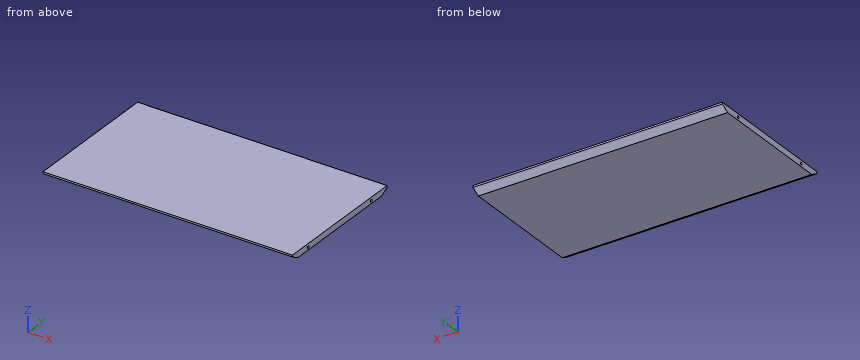
```python
from build123d import *

# Parameters (mm, degrees)
F0_W           = 800
F0_H           = 450
F1_DEPTH       = 20
F3_START       = -400.001
F3_DEPTH       = 800.002
F6_D           = 8
F6_DEPTH       = 30
F6_TIP         = 2.4034424761
F6_ON_F5_D     = 8
F6_ON_F5_DEPTH = 30
F6_ON_F5_TIP   = 2.4034424761


with BuildPart() as f1:
    # F0 (on Top) → F1 (new body)
    with BuildSketch(Plane.XY):
        Rectangle(F0_W, F0_H)
    extrude(amount=F1_DEPTH)

    # F2 (on Right) → F3 (intersect)
    with BuildSketch(Plane.YZ.offset(F3_START)):
        Polygon((-200, 0), (200, 0), (234.6410161514, 20), (-234.6410161514, 20), align=None)
    extrude(amount=F3_DEPTH, mode=Mode.INTERSECT)

    # F6
    with Locations(Plane(origin=(-400, 0, 0), x_dir=(0, -1, 0), z_dir=(-1, 0, 0))):
        with Locations((-150, 9), (150, 9)):
            Hole(F6_D / 2, depth=F6_DEPTH)
            with Locations((0, 0, -(F6_DEPTH + F6_TIP / 2))):  # 118° drill point
                Cone(0, F6_D / 2, F6_TIP, mode=Mode.SUBTRACT)

    # F6 on F5
    with Locations(Plane.YZ.offset(400)):
        with Locations((150, 9), (-150, 9)):
            Hole(F6_ON_F5_D / 2, depth=F6_ON_F5_DEPTH)
            with Locations((0, 0, -(F6_ON_F5_DEPTH + F6_ON_F5_TIP / 2))):  # 118° drill point
                Cone(0, F6_ON_F5_D / 2, F6_ON_F5_TIP, mode=Mode.SUBTRACT)


solid = f1.part
```
Verification items for the finished model (mm, model axes). Round coordinates to 2 decimals unless told otherwise and drop trailing zeros. Loops run counter-clockwise (first coordinate to the right, second up) from the corner with the lowest first, then second, coordinate; pieces in that order, holes last. Notation, with made-up numbers: (-16.75, 80) -> (39.25, 80) arc R13 cw to (39.25, 89) -> close; hole circle Ø5 at (47.5, -29). An arc over 180 degrees is marked (long way). Answer as a JSON object with one key per item and string values.
Q1. Section check A-A (x = 82.5). Record the boundary of the cut face in (y, z).
Data:
{"outline": "(-225, 14.43) -> (-200, 0) -> (200, 0) -> (225, 14.43) -> (225, 20) -> (-225, 20) -> close"}
Q2. Scan lines: line 1 (Z direction, x = 392.5, y = -150); line 2 (Y direction, x = -389.5, z = 9); line 3 (Z direction, x = -168, y = -203.5). Record each from-to range of solid material in increasing order. Write a range as from..to.
Data:
{"line 1": "z = 0..5, 13..20", "line 2": "y = -215.59..-154, -146..146, 154..215.59", "line 3": "z = 2.02..20"}
Q3. Go/stop test with flat-tipped pins: P1, Ø3, axis at x = 250, z = 11.5, coming from the +Y side; P2, Ø7, axis at y = -150, z = 9, coming from the +X side; P3, Ø6, axis at x = 195, z = 13, coming from the -Y side; P4, Ø6.5, axis at y = 150, z = 9, coming from the +X side. Record where each tip stops, or that it passes through.
Data:
{"P1": "stops at y = 222.52", "P2": "stops at x = 369.7", "P3": "stops at y = -225", "P4": "stops at x = 369.55"}
